Autodesk Inventor part; units mm, degrees
ref_plane "YZ Plane" through (0, 0, 0) normal (1, 0, 0) x (0, 1, 0)
ref_plane "XZ Plane" through (0, 0, 0) normal (0, 1, 0) x (-1, 0, 0)
ref_plane "XY Plane" through (0, 0, 0) normal (0, 0, 1) x (1, 0, 0)
sketch "Sketch2" plane through (0, 0, 0) normal (0, 0, 1) x (1, 0, 0)
  line L0 (-193.6378, 193.6378) -> (0, 273.8452)
  line L1 (0, 273.8452) -> (193.6378, 193.6378)
  line L2 (193.6378, 193.6378) -> (273.8452, 0)
  line L3 (273.8452, 0) -> (193.6378, -193.6378)
  line L4 (193.6378, -193.6378) -> (0, -273.8452)
  line L5 (0, -273.8452) -> (-193.6378, -193.6378)
  line L6 (-193.6378, -193.6378) -> (-273.8452, 0)
  line L7 (-273.8452, 0) -> (-193.6378, 193.6378)
  circle A0 centre (0, 0) radius 180
  dimension "d23" = 506
  dimension "d26" = 360
extrude "Plate1" add sketch "Sketch2" against normal blind 3
sketch "Sketch4" plane through (0, 0, 0) normal (0, 0, 1) x (1, 0, 0)
  circle A0 centre (0, 200) radius 6.25
  circle A1 centre (0, 0) radius 180
  dimension "d16" = 12.5
  dimension "d17" = 200
extrude "Extrusion1" cut sketch "Sketch4" against normal up to surface (3 mm away) contours A0
pattern_circular "Circular Pattern1" count 8 over 360 about axis through (0, 0, -10) along (0, 0, 1) of "Extrusion1"
equation "\"d23\" = Барабан_габарит_по_кассетам"
equation "\"d26\" = Вал_ось_диаметр_КОРМА"
equation "\"d15\" = Thickness"
equation "\"BendRadius\" = Thickness"
equation "\"BendReliefWidth\" = Thickness"
equation "\"BendReliefDepth\" = 0.5 * Thickness"
equation "\"CornerReliefSize\" = 4 * Thickness"
equation "\"MinimumRemnant\" = 2 * Thickness"
equation "\"TransitionRadius\" = BendRadius"
equation "\"JacobiRadiusSize\" = BendRadius"
equation "\"GapSize\" = Thickness"
properties part number "ДМС 101 Барабан торец зад"
Can you work these out from the model? Positions are in its coordinate system, mm. Give positions to 0.01 mm unless a question says otherwise; leave off trailing zeros. Loops run counter-clockwise (first coordinate to the right, second up) from the corner with the lowest first, then second, coordinate; pieces in that order, holes last. Notation, with made-up numbers: M 59,66 L 101,66 A24 ccw 101,86 Z; hole C 42.25,0.25 d2. An arc over 180 degrees is marked long. One line per item, written item: value.
1) Imagine slicing it at C-C on z = -0.7. Count the separate pieces of the cut face and the enclosed holes in it, and give its area (3 significant figures).
Geometry check:
separate pieces: 1
enclosed holes: 9
area: 109,000 mm²
2) Imagine slicing it at A-A on x = 45. Write out the boundary of the cut face in (y, z).
Geometry check:
outline: M -255.21,-3 L -174.28,-3 L -174.28,0 L -255.21,0 Z; M 174.28,-3 L 255.21,-3 L 255.21,0 L 174.28,0 Z
3) Imagine slicing it at D-D on y = -214. Write out the boundary of the cut face in (x, z), and give its area (3 significant figures).
Geometry check:
outline: M -144.48,-3 L 144.48,-3 L 144.48,0 L -144.48,0 Z
area: 867 mm²
4) Thinking about a two-plate mould opening in Y: for faces 1 (the face through (-194.455, 2.884, -1.479)), 2 (the face through (234.303, -95.463, -1.479)), 3 (the face through (-4, 186, -3)), which applies, +Y half, -Y half, draft (parallel to the pull), parting line (faces both ways), or undercut?
Geometry check:
face 1: undercut
face 2: -Y half
face 3: draft
5) I'm going to push a flat-ended pin straight in: pin 1 (1 mm diameter, centred on y = -118, z = -1.5, fed in from -X). Where does the tip first touch, or does it pass through?
Geometry check:
pin 1: stops at x = -225.18
6) Imagine slicing it at B-B on y = 127.5. Write out the boundary of the cut face in (x, z).
Geometry check:
outline: M -221.03,-3 L -127.06,-3 L -127.06,0 L -221.03,0 Z; M 127.06,-3 L 221.03,-3 L 221.03,0 L 127.06,0 Z
7) Please list where these lines run through material, in increasing order: line 1 (Y direction, x = 0, z = -2.4); line 2 (X direction, y = -90, z = -2.05); line 3 (Y direction, x = 112, z = -2.75).
Geometry check:
line 1: y = -273.85 to -206.25, -193.75 to -180, 180 to 193.75, 206.25 to 273.85
line 2: x = -236.57 to -155.88, 155.88 to 236.57
line 3: y = -227.45 to -140.91, 140.91 to 227.45
